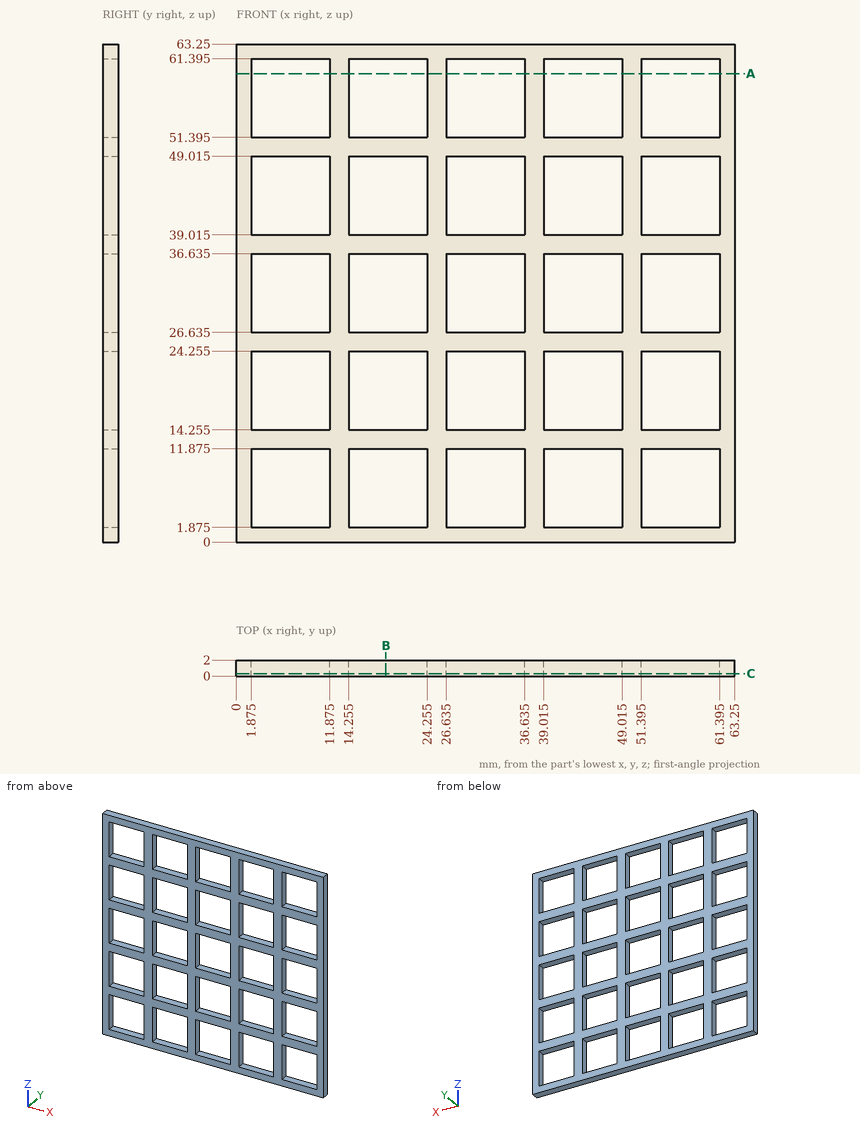
For this review, use the dimensioned drawing (mm, ordinates from the lowest corner) and the shaded views. Give positions to 0.01 mm unless a question says otherwise; leave off trailing zeros. Write each loop counter-clockwise with the first axis right and the second up, starting at its lowest first coordinate (ties: lowest second). Pieces come first, ordered by that corner, then holes. Notation, with made-up numbers: M 2,60.25 L 13,60.25 A17 cw 13,91.25 Z; hole C 73,-31.75 d5. An arc over 180 degrees is marked long. Write item = value, one per line. Start each with the question number.
Q1. We need section A-A (z = 59.5). State the section outline as (x, y) points (3 decimals).
Q2. We need section B-B (x = 19). State the section outline as (y, z) points (3 decimals).
Q3. We need section C-C (y = 0.3). Give the number of separate pieces and of enclosed holes in the cut face, plus the area to 3 significant figures.
Q4. For line 1 (X direction, y = 0.55, z = 60) (3 decimals), list the stretches that pass through material, from the lowest coordinate up.
Result set:
q1.outline = M 0,0 L 1.875,0 L 1.875,2 L 0,2 Z; M 11.875,0 L 14.255,0 L 14.255,2 L 11.875,2 Z; M 24.255,0 L 26.635,0 L 26.635,2 L 24.255,2 Z; M 36.635,0 L 39.015,0 L 39.015,2 L 36.635,2 Z; M 49.015,0 L 51.395,0 L 51.395,2 L 49.015,2 Z; M 61.395,0 L 63.25,0 L 63.25,2 L 61.395,2 Z
q2.outline = M 0,0 L 2,0 L 2,1.875 L 0,1.875 Z; M 0,11.875 L 2,11.875 L 2,14.255 L 0,14.255 Z; M 0,24.255 L 2,24.255 L 2,26.635 L 0,26.635 Z; M 0,36.635 L 2,36.635 L 2,39.015 L 0,39.015 Z; M 0,49.015 L 2,49.015 L 2,51.395 L 0,51.395 Z; M 0,61.395 L 2,61.395 L 2,63.25 L 0,63.25 Z
q3.separate_pieces = 1
q3.enclosed_holes = 25
q3.area = 1,500 mm2
q4.line_1 = 0 to 1.875, 11.875 to 14.255, 24.255 to 26.635, 36.635 to 39.015, 49.015 to 51.395, 61.395 to 63.25
